Autodesk Inventor part; units mm, degrees
ref_plane "YZ Plane" through (0, 0, 0) normal (1, 0, 0) x (0, 1, 0)
ref_plane "XZ Plane" through (0, 0, 0) normal (0, 1, 0) x (-1, 0, 0)
ref_plane "XY Plane" through (0, 0, 0) normal (0, 0, 1) x (1, 0, 0)
sketch "Sketch1" plane through (0, 0, 0) normal (0, 1, 0) x (-1, 0, 0)
  line L0 (103.6486, 142.7027) -> (-186.3514, 142.7027)
  line L1 (-186.3514, 142.7027) -> (-186.3514, -17.2973)
  line L2 (103.6486, -17.2973) -> (103.6486, 142.7027)
  circle A0 centre (-41.3514, 138.2027) radius 1
  circle A1 centre (-41.3514, 122.2027) radius 1
  circle A2 centre (-33.3514, 130.2027) radius 1
  circle A3 centre (-49.3514, 130.2027) radius 1
  line L3 (-186.3514, -17.2973) -> (-71.3514, -17.2973)
  line L4 (-71.3514, -17.2973) -> (-71.3514, 62.7027)
  line L5 (-71.3514, 62.7027) -> (-11.3514, 62.7027)
  line L6 (-11.3514, 62.7027) -> (-11.3514, -17.2973)
  line L7 (-11.3514, -17.2973) -> (103.6486, -17.2973)
  point P0 (0, 0)
  dimension "d0" = 290
  dimension "d1" = 160
  dimension "d2" = 4.5
  dimension "d3" = 2
  dimension "d5" = 2
  dimension "d6" = 16
  dimension "d8" = 2
  dimension "d9" = 2
  dimension "d10" = 8
  dimension "d11" = 8
  dimension "d12" = 8
  dimension "d13" = 8
  dimension "d16" = 145
  dimension "d17" = 145
  dimension "d18" = 60
  dimension "d19" = 115
  dimension "d20" = 80
extrude "Extrusion1" add sketch "Sketch1" along normal blind 5
properties part number "etage_support_minerai"
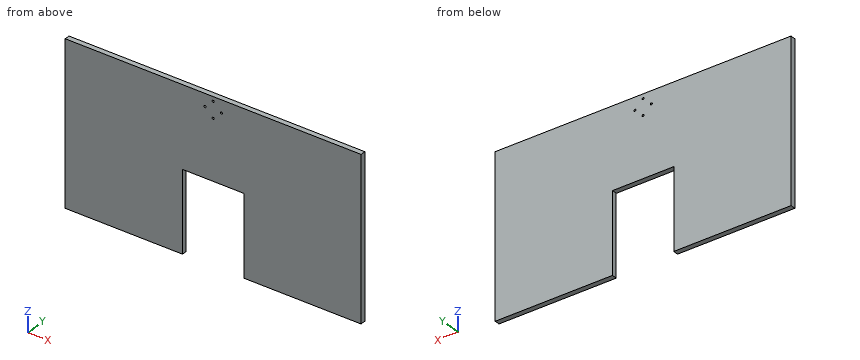
Work out the finished part from the listing and answer in its coordinate system (mm). Coordinates: 2 decimals unless noted, no trailing zeros. Write each loop counter-clockwise with the first axis right and the second up, starting at its lowest first coordinate (ties: lowest second). Pieces come first, ordered by that corner, then holes.
1. The part is cut by section A-A, the plane z = 13. Write down the section's boundary in (x, y).
Results list:
outline: (-103.65, 0) - (11.35, 0) - (11.35, 5) - (-103.65, 5) - close; (71.35, 0) - (186.35, 0) - (186.35, 5) - (71.35, 5) - close
2. A flat-ended cylindrical pin translates along its axis: pin 1 (2.5 mm diameter, centred on x = 41.35, z = 138.2, fed in from +Y). Find the tip coordinate at first contact, or state that the pin passes through.
Results list:
pin 1: stops at y = 5
3. Consider line 1 along X through (y, z) = (3.7, 33.5); line 2 along Z through (x, y) = (68.5, 4.6). Determine where each line is inside the solid, lowest interval first.
Results list:
line 1: x = -103.65 to 11.35, 71.35 to 186.35
line 2: z = 62.7 to 142.7
4. The part is cut by section B-B, the plane y = 3.75. Write down the section's boundary in (x, z), and give its area (3 significant figures).
Results list:
outline: (-103.65, -17.3) - (11.35, -17.3) - (11.35, 62.7) - (71.35, 62.7) - (71.35, -17.3) - (186.35, -17.3) - (186.35, 142.7) - (-103.65, 142.7) - close; hole circle Ø2 at (33.35, 130.2); hole circle Ø2 at (41.35, 122.2); hole circle Ø2 at (41.35, 138.2); hole circle Ø2 at (49.35, 130.2)
area: 41,600 mm2
